Part print with two shaded views. Sizes in mm from the minimum x, y, z corner. Round coordinates to 2 decimals unless told otherwise and drop trailing zeros. Order: outer loops, then holes, each group sorted by start corner. A loop starts at its lowest first (then second) coordinate and runs counter-clockwise, first axis right, second up. Notation, with made-up numbers: (46.25, 38) - (56.25, 38) arc R16 cw to (56.25, 55) - close; hole circle Ø7 at (-27, -31). An arc over 180 degrees is marked (long way). Answer as CSV lines item,"result". Start each with the question number.
1. Wall check: line 1 along Y through (x, z) = (12.7, 24.05); line 2 along Y through (x, z) = (14, 23). Give the ranges that are in metal, low to high. Write a range as [from, to].
2. Band-saw the part on A-A on x = 12.7. List the corners of the cut face in (y, z).
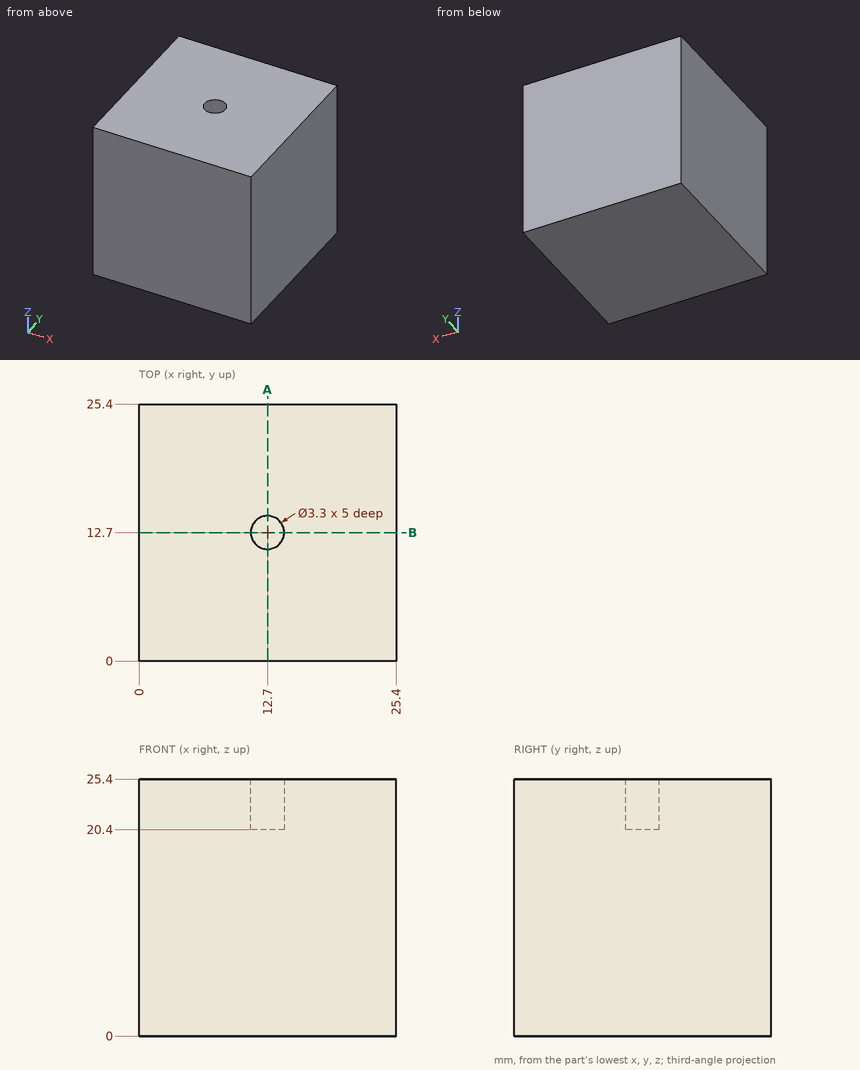
Reply:
1,line 1,"y = [0, 11.05], [14.35, 25.4]"
1,line 2,"y = [0, 11.68], [13.72, 25.4]"
2,outline,"(0, 0) - (25.4, 0) - (25.4, 25.4) - (14.35, 25.4) - (14.35, 20.4) - (11.05, 20.4) - (11.05, 25.4) - (0, 25.4) - close"
